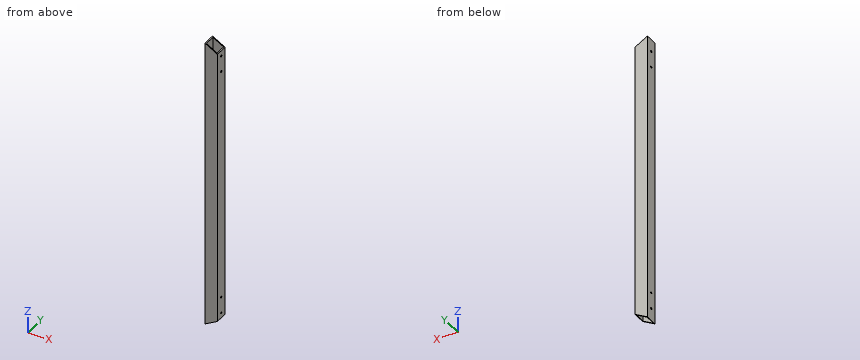
```python
from build123d import *

# Parameters (mm, degrees)
SKETCH1_W           = 44.45
SKETCH1_H           = 44.45
SKETCH1_W_2         = 38.1
SKETCH1_H_2         = 38.1
BOSS_EXTRUDE1_DEPTH = 1041.4
CUT_EXTRUDE2_DEPTH  = 1041.4
SKETCH9_R           = 3.3734375
CUT_EXTRUDE3_DEPTH  = 1043.585110734


with BuildPart() as part:
    # Sketch1 → Boss-Extrude1 (new body)
    with BuildSketch(Plane.XY):
        Rectangle(SKETCH1_W, SKETCH1_H)
        Rectangle(SKETCH1_W_2, SKETCH1_H_2, mode=Mode.SUBTRACT)
    extrude(amount=BOSS_EXTRUDE1_DEPTH)

    # Sketch2 → Cut-Extrude2 (cut)
    with BuildSketch(Plane(origin=(0, 22.225, 0), x_dir=(1, 0, 0), z_dir=(0, 1, 0))):
        Polygon((-22.225, -1041.4), (22.225, -1041.4), (22.225, -1015.736780535), align=None)
        Polygon((-22.225, 0), (22.225, -25.663219465), (22.225, 0), align=None)
    extrude(amount=-CUT_EXTRUDE2_DEPTH, mode=Mode.SUBTRACT)

    # Sketch9 → Cut-Extrude3 (cut, through all)
    with BuildSketch(Plane.ZY.offset(22.225)):
        with Locations((996.95, 0)):
            Circle(SKETCH9_R)
        with Locations((44.45, 0)):
            Circle(SKETCH9_R)
        with Locations((102.389658314, 0)):
            Circle(SKETCH9_R)
        with Locations((939.010341686, 0)):
            Circle(SKETCH9_R)
    extrude(amount=-CUT_EXTRUDE3_DEPTH, mode=Mode.SUBTRACT)


solid = part.part
```
Model file for the job. Use its own axes, mm. Give positions to 0.01 mm unless a question says otherwise; leave off trailing zeros. Loops run counter-clockwise (first coordinate to the right, second up) from the corner with the lowest first, then second, coordinate; pieces in that order, holes last. Notation, with made-up numbers: (-32.5, 69.5) -> (9.5, 69.5) arc R25 cw to (9.5, 98.5) -> close; hole circle Ø11 at (38.5, -6.75). An arc over 180 degrees is marked (long way). Use CSV: the item, a comma, the result in double quotes. Start each with the question number.
1) Slice it at C-C on x = 10.5. Give the cut face in (y, z) (3 decimals), plus the area to 3 significant figures.
2) Slice it at B-B on z = 819. Give the cut face in (x, y) (3 decimals), plus the area to 3 significant figures.
3) Flat gauge pins, fed straight in: pin 1 Ø5.5 at (y, z) = (0, 939.01) entering from -X; pin 2 Ø10 at (x, y) = (-14.5, -8) entering from +Z. Where does each tip first touch, or does it go through?
4) Wall check: line 1 (X direction, y = 17, z = 998.5) (3 decimals). Give the ranges that are in metal, low to high.
5) Slice it at A-A on y = -12. Give the cut face in (x, z) (3 decimals), plus the area to 3 significant figures.
Computed values:
1,outline,"(-22.225, 18.894) -> (-19.05, 18.894) -> (-19.05, 1022.506) -> (-22.225, 1022.506) -> close; (19.05, 18.894) -> (22.225, 18.894) -> (22.225, 1022.506) -> (19.05, 1022.506) -> close"
1,area,"6,370 mm^2"
2,outline,"(-22.225, -22.225) -> (22.225, -22.225) -> (22.225, 22.225) -> (-22.225, 22.225) -> close; hole (-19.05, -19.05) -> (19.05, -19.05) -> (19.05, 19.05) -> (-19.05, 19.05) -> close"
2,area,"524 mm^2"
3,pin 1,"passes through"
3,pin 2,"stops at z = 1039.83"
4,line 1,"x = -22.225 to -19.05, 19.05 to 22.225"
5,outline,"(-22.225, 0) -> (-19.05, 1.833) -> (-19.05, 1039.567) -> (-22.225, 1041.4) -> close; (19.05, 23.83) -> (22.225, 25.663) -> (22.225, 1015.737) -> (19.05, 1017.57) -> close"
5,area,"6,450 mm^2"
